Read the model definition and answer for the solid it produces. Units are mm, in the model's axes. Face numbers are marked on the shaded views. Coordinates: 2 decimals unless noted, no trailing zeros. Order: outer loops, then holes, each group sorted by start corner. A loop starts at its lowest first (then second) coordinate and runs counter-clockwise, first axis right, second up. Notation, with made-up numbers: M 72.5,-10 L 115.5,-10 A8 ccw 115.5,-2 Z; hole C 59,22.25 d5. An arc over 180 degrees is marked long. One line per question, with ' | ' between items. Start each with the question number.
1) Given P1, Ø1.8, axis at x = -20, y = 25.5, coming from the -Z side; P2, Ø3, axis at y = 8.5, z = 12.5, coming from the +X side; P3, Ø1.9, axis at y = 23, z = 18, coming from the +X side, each flat-ended and moving along its own axis, determine where each tip first touches the part or whether it passes through.
2) Find section C-C, the plane x = 11. Write down the section's boundary in (y, z).
3) The mould has two halves that part along X. Classify the marked faces 1, 2 and 3: +X half, -X half, draft (parallel to the pull), parting line (faces both ways), or undercut.
4) Find section D-D, the plane z = 15. Write down the section's boundary in (x, y), plus the area to 3 significant figures.
5) Find section A-A, the plane y = 36.5. Write down the section's boundary in (x, z), plus the area to 3 significant figures.
6) Consider probe 1 along X at (y, z) = (38, 19.75); probe 2 along Y at (x, z) = (10, 1); probe 3 along X at (y, z) = (22, 16.5). Determine where each line is inside the solid, lowest interval first.
7) Find section B-B, the plane z = 7. Write down the section's boundary in (x, y).
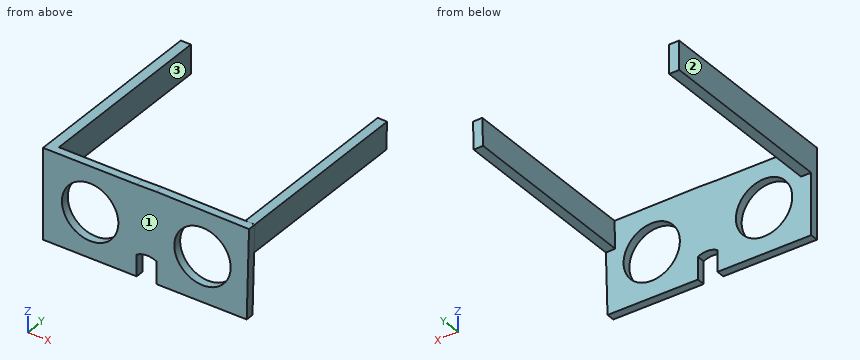
from build123d import *

# Parameters (mm, degrees)
F0_R     = 9.7397478584
F0_R_2   = 9.242675957
F1_DEPTH = 1.8415
F2_D     = 12.7
F4_W     = 41.9321846507
F4_H     = 6.4849769697
F5_DEPTH = 2.286
F3_W     = 41.9973064504
F3_H     = 6.2387038374
F6_DEPTH = 2.0955


# Not quite as in the source:
# - a feature names something its author has since deleted; it is built from what else it names


with BuildPart() as f1:
    # F0 (on Front) → F1 (new body)
    with BuildSketch(Plane.XZ):
        with BuildLine():
            Line((0, 4.8052047364), (0, 20.2608313411))
            Line((0, 20.2608313411), (-21.113075316, 20.2608313411))
            Line((-21.113075316, 20.2608313411), (-21.113075316, 0))
            Line((-21.113075316, 0), (-2.0606040489, 0))
            ThreePointArc((-2.0606040489, 0), (-1.7849391427, 2.7262115351), (0, 4.8052047364))
        make_face()
        with Locations((-10.4878218845, 10.1304156706)):
            Circle(F0_R, mode=Mode.SUBTRACT)
        with BuildLine():
            Line((25.3197303883, 20.1294401959), (4.4281314508, 20.3600343892))
            Line((4.4281314508, 20.3600343892), (4.4281314508, 19.6842234582))
            Line((4.4281314508, 19.6842234582), (4.4281314508, 5.0302978839))
            ThreePointArc((4.4281314508, 5.0302978839), (6.5221702803, 2.937211036), (6.8947323598, 0))
            Line((6.8947323598, 0), (24.7934444089, 0))
            Line((24.7934444089, 0), (25.3197303883, 20.1294401959))
        make_face()
        with Locations((14.8297464475, 10.0766858086)):
            Circle(F0_R_2, mode=Mode.SUBTRACT)
        with Locations((-10.4878218845, 10.1304156706)):
            Circle(F0_R)
        with Locations((14.8297464475, 10.0766858086)):
            Circle(F0_R_2)
        with BuildLine():
            Line((4.4281314508, 20.3600343892), (0, 20.2608313411))
            Line((0, 20.2608313411), (0, 4.8052047364))
            ThreePointArc((0, 4.8052047364), (2.1849540655, 5.490448695), (4.4281314508, 5.0302978839))
            Line((4.4281314508, 5.0302978839), (4.4281314508, 19.6842234582))
            Line((4.4281314508, 19.6842234582), (4.4281314508, 20.3600343892))
        make_face()
        with BuildLine():
            ThreePointArc((6.8947323598, 0), (6.5221702803, 2.937211036), (4.4281314508, 5.0302978839))
            Line((4.4281314508, 5.0302978839), (4.4281314508, 0))
            Line((4.4281314508, 0), (6.8947323598, 0))
        make_face()
        with BuildLine():
            Line((0, 0), (0, 4.8052047364))
            ThreePointArc((0, 4.8052047364), (-1.7849391427, 2.7262115351), (-2.0606040489, 0))
            Line((-2.0606040489, 0), (0, 0))
        make_face()
    extrude(amount=-F1_DEPTH)

    # F2 (through all)
    with Locations(Plane.XZ):
        with Locations((-10.4878218845, 10.1304156706), (14.8297464475, 10.0766858086)):
            Hole(F2_D / 2)

    # F4 (on face) → F5 (join)
    with BuildSketch(Plane(origin=(-21.113075316, 0, 0), x_dir=(0, -1, 0), z_dir=(-1, 0, 0))):
        with Locations((-22.8075923253, 17.0183428563)):
            Rectangle(F4_W, F4_H)
    extrude(amount=-F5_DEPTH)

    # F3 (on face) → F6 (join)
    with BuildSketch(Plane(origin=(24.77650804, 0, -0.6477839757), x_dir=(0, 1, 0), z_dir=(0.9996583923, 0, -0.0261361563))):
        with Locations((22.8401532252, 17.6649723378)):
            Rectangle(F3_W, F3_H)
    extrude(amount=-F6_DEPTH)


solid = f1.part
Report:
1) P1: stops at z = 13.78 | P2: stops at x = 25.16 | P3: stops at x = 25.29
2) outline: M 0,0 L 1.84,0 L 1.84,5.01 L 0,5.01 Z; M 0,15.14 L 1.84,15.14 L 1.84,20.29 L 0,20.29 Z
3) face 1: draft | face 2: -X half | face 3: undercut
4) outline: M -21.11,0 L -14.56,0 L -14.56,1.84 L -18.83,1.84 L -18.83,43.77 L -21.11,43.77 Z; M -6.41,0 L 10.82,0 L 10.82,1.84 L -6.41,1.84 Z; M 18.84,0 L 25.19,0 L 25.19,43.84 L 23.09,43.84 L 23.09,1.84 L 18.84,1.84 Z | area: 239 mm^2
5) outline: M -21.11,13.78 L -18.83,13.78 L -18.83,20.26 L -21.11,20.26 Z; M 23.06,13.95 L 25.16,13.89 L 25.32,20.13 L 23.22,20.18 Z | area: 27.9 mm^2
6) probe 1: x = -21.11 to -18.83, 23.21 to 25.31 | probe 2: y = 0 to 1.84 | probe 3: x = -21.11 to -18.83, 23.13 to 25.22
7) outline: M -21.11,0 L -16.01,0 L -16.01,1.84 L -21.11,1.84 Z; M -4.96,0 L 9.27,0 L 9.27,1.84 L -4.96,1.84 Z; M 20.38,0 L 24.98,0 L 24.98,1.84 L 20.38,1.84 Z
